from build123d import *

# Parameters (mm, degrees)
SKETCH_W               = 47.7
SKETCH_H               = 23.7
PAD_DEPTH              = 14.4
SKETCH001_W            = 44.1
SKETCH001_H            = 20.1
POCKET_DEPTH           = 12.6
SKETCH002_R            = 3.6
PAD001_DEPTH           = 2.7
LINEARPATTERN_COUNT    = 4
LINEARPATTERN_PITCH    = 12
SKETCH003_R            = 4.8825
PAD002_DEPTH           = 12.6
LINEARPATTERN001_COUNT = 3
LINEARPATTERN001_PITCH = 12
SKETCH004_R            = 3.6
POCKET001_DEPTH        = 12.6
LINEARPATTERN002_COUNT = 3
LINEARPATTERN002_PITCH = 12


with BuildPart() as part:
    # Sketch → Pad (new body)
    with BuildSketch(Plane.XY):
        with Locations((23.85, -11.85)):
            Rectangle(SKETCH_W, SKETCH_H)
    extrude(amount=PAD_DEPTH)

    # Sketch001 (on Face5 of Pad) → Pocket (cut)
    with BuildSketch(Plane(origin=(0, 0, 0), x_dir=(1, 0, 0), z_dir=(0, 0, -1))):
        with Locations((23.85, 11.85)):
            Rectangle(SKETCH001_W, SKETCH001_H)
    extrude(amount=-POCKET_DEPTH, mode=Mode.SUBTRACT)

    # Sketch002 (on Face5 of Pocket) → Pad001 (join)
    with BuildSketch(Plane.XY.offset(14.4)):
        with Locations((6, -6)):
            Circle(SKETCH002_R)
        with Locations((6, -17.7)):
            Circle(SKETCH002_R)
    pad001 = extrude(amount=PAD001_DEPTH)

    # LinearPattern: Pad001 ×4
    with Locations(*[(i * LINEARPATTERN_PITCH, 0, 0) for i in range(1, LINEARPATTERN_COUNT)]):
        add(pad001)

    # Sketch003 (on Face19 of LinearPattern) → Pad002 (join)
    with BuildSketch(Plane(origin=(0, 0, 12.6), x_dir=(1, 0, 0), z_dir=(0, 0, -1))):
        with Locations((12, 12)):
            Circle(SKETCH003_R)
    pad002 = extrude(amount=PAD002_DEPTH)

    # LinearPattern001: Pad002 ×3
    with Locations(*[(i * LINEARPATTERN001_PITCH, 0, 0) for i in range(1, LINEARPATTERN001_COUNT)]):
        add(pad002)

    # Sketch004 (on Face31 of LinearPattern001) → Pocket001 (cut)
    with BuildSketch(Plane(origin=(0, 0, 0), x_dir=(1, 0, 0), z_dir=(0, 0, -1))):
        with Locations((12, 12)):
            Circle(SKETCH004_R)
    pocket001 = extrude(amount=-POCKET001_DEPTH, mode=Mode.SUBTRACT)

    # LinearPattern002: Pocket001 ×3
    with Locations(*[(i * LINEARPATTERN002_PITCH, 0, 0) for i in range(1, LINEARPATTERN002_COUNT)]):
        add(pocket001, mode=Mode.SUBTRACT)


solid = part.part
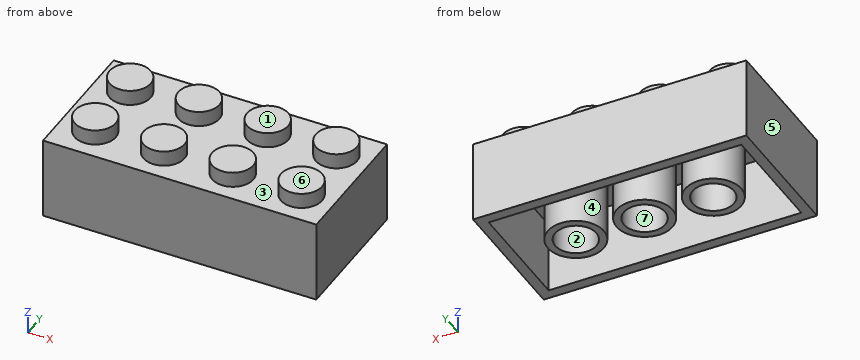
CAD build for the part. Positions are in the model's coordinates, mm. Face numbers are marked on the shaded views. A direction names the side the tool comes from. Round coordinates to 2 decimals unless told otherwise and drop trailing zeros. Write each loop counter-clockwise with the first axis right and the second up, starting at its lowest first coordinate (ties: lowest second). Pieces come first, ordered by that corner, then holes. Notation, with made-up numbers: M 30,-9 L 50,-9 A11 ccw 50,9 Z; hole C 26.5,40.25 d6. An arc over 180 degrees is marked long. Put each result on its own line as item: value. Start each with the question number.
1) Saw through at A-A, the plane z = 4.5. Write the cut outline in (x, y) (1 decimal), and give its area (3 significant figures).
2) Pin check, flat tips, straight feed: pin 1 Ø4.5 at (x, y) = (24, -12) entering from +Z; pin 2 Ø2 at (x, y) = (23, -11.5) entering from -Z. Stop position of each tip, or through.
3) 3-axis set-ups, long thin cutter, end or side, ignore diameter. For the marked faces 1, 2 and 3: which of +Z, -Z, +X, -X, +Y, -Y reach the whole face in a straight line?
4) Drill centre lines: probe 1 along Y at (x, z) = (24, 3); probe 2 along Y at (x, z) = (7.5, 6.75); probe 3 along X at (y, z) = (-6.25, 6.5). Where is each one in solid material? Low to high. Write a range as [from, to].
5) Saw through at B-B, the plane x = 36. Write the cut outline in (y, z).
6) Saw through at C-C, the plane y = -6. Write the cut outline in (x, z).
7) Saw through at D-D, the plane x = 6. Write the cut outline in (y, z).
8) Pull direction X, two halves, no side cores. Call the marked faces 4, 5, 6 and 7: pulls with the +X half, pulls with the -X half, needs draft (parallel to the pull), parting line crosses it, or undercut.
Resolved:
1. outline: M 0,-23.7 L 47.7,-23.7 L 47.7,0 L 0,0 Z; C 12,-12 d9.8; C 24,-12 d9.8; C 36,-12 d9.8; hole M 1.8,-21.9 L 45.9,-21.9 L 45.9,-1.8 L 1.8,-1.8 Z; hole C 12,-12 d7.2; hole C 24,-12 d7.2; hole C 36,-12 d7.2
1. area: 347 mm²
2. pin 1: z = 14.4
2. pin 2: z = 12.6
3. face 1: +Z, +X, -X, +Y, -Y
3. face 2: -Z
3. face 3: +Z
4. probe 1: [-23.7, -21.9], [-16.88, -15.6], [-8.4, -7.12], [-1.8, 0]
4. probe 2: [-23.7, -21.9], [-13.89, -10.11], [-1.8, 0]
4. probe 3: [0, 1.8], [45.9, 47.7]
5. outline: M -23.7,0 L -21.9,0 L -21.9,12.6 L -16.88,12.6 L -16.88,0 L -15.6,0 L -15.6,12.6 L -8.4,12.6 L -8.4,0 L -7.12,0 L -7.12,12.6 L -1.8,12.6 L -1.8,0 L 0,0 L 0,14.4 L -23.7,14.4 Z
6. outline: M 0,0 L 1.8,0 L 1.8,12.6 L 45.9,12.6 L 45.9,0 L 47.7,0 L 47.7,14.4 L 45.6,14.4 L 45.6,17.1 L 38.4,17.1 L 38.4,14.4 L 33.6,14.4 L 33.6,17.1 L 26.4,17.1 L 26.4,14.4 L 21.6,14.4 L 21.6,17.1 L 14.4,17.1 L 14.4,14.4 L 9.6,14.4 L 9.6,17.1 L 2.4,17.1 L 2.4,14.4 L 0,14.4 Z
7. outline: M -23.7,0 L -21.9,0 L -21.9,12.6 L -1.8,12.6 L -1.8,0 L 0,0 L 0,14.4 L -2.4,14.4 L -2.4,17.1 L -9.6,17.1 L -9.6,14.4 L -14.1,14.4 L -14.1,17.1 L -21.3,17.1 L -21.3,14.4 L -23.7,14.4 Z
8. face 4: undercut
8. face 5: pulls with the -X half
8. face 6: needs draft
8. face 7: undercut
